Model file for the job. Use its own axes, mm. A direction names the side the tool comes from. Give positions to 0.01 mm unless a question says otherwise; leave off trailing zeros. Loops run counter-clockwise (first coordinate to the right, second up) from the corner with the lowest first, then second, coordinate; pieces in that order, holes last. Notation, with made-up numbers: (-3, 70.5) - (54, 70.5) arc R19 cw to (54, 82.5) - close; hole circle Ø8 at (-25.5, 33). An arc over 180 degrees is marked (long way). Answer as CSV lines item,"result". Start each with the question number.
Item 1: Pull direction Y, two halves, no side cores. Call faces 1 (the flat face through (-20.3, 0, 7)), 2 (the flat face through (0, 15.4, 26)), 3 (the flat face through (0.148, -6.034, 30.325)): pulls with the +Y half, pulls with the -Y half, needs draft (parallel to the pull), parting line crosses it, or undercut.
Item 2: Saw through at A-A on z = 36. Give the cut face in (x, y).
Item 3: Drill centre lines: L1, parallel to X at y = -4, z = 8; L2, parallel to Y at x = 0.5, z = 28.5; L3, parallel to Z at x = 3, y = -5. Where is each one in solid material? Low to high. Write a range as from..to.
Item 4: Saw through at D-D on x = 7.5. Give the cut face in (y, z).
Item 5: Pin check, flat tips, straight feed: pin 1 (1.7 mm diameter, centred on x = -18, z = 15.5, fed in from +Y); pin 2 (1.5 mm diameter, centred on y = 5.5, z = 34.5, fed in from -X); pin 3 (10 mm diameter, centred on x = 12.5, z = 30.5, fed in from +Y); pin 4 (2 mm diameter, centred on y = -9, z = 23, fed in from +X). Stop position of each tip, or through.
Item 6: Tool access for faces 4 (the flat face through (18, -9.4, 8)), 5 (the flat face through (-18, 0, 0)), 6 (the flat face through (-10.6, 0, 30)): list every direction of +Z, -Z, +X, -X, +Y, -Y with a clear straight run to the whole face (end or side of a thin tool).
Item 7: Saw through at B-B on z = 7.5. Give the cut face in (x, y), plus the area to 3 significant figures.
Autodesk Inventor part; units mm, degrees
ref_plane "YZ Plane" through (0, 0, 0) normal (1, 0, 0) x (0, 1, 0)
ref_plane "XZ Plane" through (0, 0, 0) normal (0, 1, 0) x (-1, 0, 0)
ref_plane "XY Plane" through (0, 0, 0) normal (0, 0, 1) x (1, 0, 0)
sketch "Sketch1" plane through (0, 0, 0) normal (0, 0, 1) x (1, 0, 0)
  line L0 (-20.3, 9.4) -> (20.3, 9.4)
  line L1 (20.3, 9.4) -> (20.3, -9.4)
  line L2 (20.3, -9.4) -> (-20.3, -9.4)
  line L3 (-20.3, -9.4) -> (-20.3, 9.4)
  line L4 (-14.7, 9.4) -> (14.7, 9.4)
  line L5 (14.7, 9.4) -> (14.7, -9.4)
  line L6 (14.7, -9.4) -> (-14.7, -9.4)
  line L7 (-14.7, -9.4) -> (-14.7, 9.4)
  point P0 (0, 0)
  point P1 (14.7, 9.4)
  dimension "d0" = 29.4
  dimension "d1" = 18.8
  dimension "d2" = 9.4
  dimension "d3" = 14.7
  dimension "d4" = 5.6
  dimension "d5" = 5.6
extrude "Extrusion1" add sketch "Sketch1" along normal blind 18
extrude "Extrusion2" cut sketch "Sketch1" along normal blind 10 contours L0 L5 L2 L7
sketch "Sketch2" plane through (0, 0, 18) normal (0, 0, 1) x (1, 0, 0)
  line L0 (10.6, 0) -> (-10.6, 12.2398)
  line L1 (-10.6, 12.2398) -> (-10.6, -12.2398)
  line L2 (14.7, 9.4) -> (-14.7, 9.4)
  line L3 (-10.6, -12.2398) -> (10.6, 0)
  line L4 (-20.3, 9.4) -> (-20.3, -9.4)
  line L5 (14.7, -9.4) -> (14.7, 9.4)
  line L6 (-14.7, 9.4) -> (-14.7, -9.4)
  line L7 (14.7, -9.4) -> (-14.7, -9.4)
  line L8 (-14.7, -9.4) -> (-14.7, -15.4)
  line L9 (-14.7, -15.4) -> (14.7, -15.4)
  line L10 (14.7, -15.4) -> (14.7, -9.4)
  line L11 (14.7, 9.4) -> (-14.7, 9.4)
  line L12 (-14.7, 9.4) -> (-14.7, 15.4)
  line L13 (-14.7, 15.4) -> (14.7, 15.4)
  line L14 (14.7, 15.4) -> (14.7, 9.4)
  point P0 (0, 0)
  point P1 (-10.6, 0)
  point P2 (0, -6.1199)
  point P3 (0, 6.1199)
  point P4 (-14.7, 9.4)
  point P5 (-14.7, -9.4)
  point P6 (-5.6813, -9.4)
  point P7 (-10.6, -9.4)
  point P8 (-10.6, 9.4)
  point P9 (-5.6813, 9.4)
  dimension "d17" = 21.2
  dimension "d18" = 0
  dimension "d19" = 21.2
  dimension "d20" = 21.2
  dimension "d21" = 10.6
  dimension "d25" = 6
  dimension "d26" = 6
  dimension "d27" = 0
  dimension "d28" = 0
extrude "Extrusion3" add sketch "Sketch2" along normal blind 10 and the other way blind 8 contours L0 L2 L5 L7 L3 | L0 L1 L2 L12 L13 L14 | L7 L10 L9 L8 L1 L3 | L1 L7 L6 L2
extrude "Extrusion4" add sketch "Sketch2" against normal blind 8 contours L2 L1 L0 | L3 L1 L7
chamfer "Chamfer1" distance 6 angle 45 4 edges at (-14.7, 15.4, 19) (-14.7, -15.4, 19) (14.7, -15.4, 19) (14.7, 15.4, 19)
fillet "Fillet1" radius 3 4 edges at (14.7, 0, 18) (-14.7, 0, 18) (-20.3, 0, 18) (20.3, 0, 18)
sketch "Sketch4" plane through (0, 0, 28) normal (0, 0, 1) x (1, 0, 0)
  line L0 (8.7, 15.4) -> (14.7, 9.4)
  line L1 (8.7, 15.4) -> (-8.7, 15.4)
  line L2 (-14.7, 9.4) -> (-8.7, 15.4)
  line L3 (-14.7, 9.4) -> (-14.7, -9.4)
  line L4 (-8.7, -15.4) -> (-14.7, -9.4)
  line L5 (-8.7, -15.4) -> (8.7, -15.4)
  line L6 (14.7, -9.4) -> (8.7, -15.4)
  line L7 (14.7, -9.4) -> (14.7, 9.4)
  line L8 (-10.6, 12.2398) -> (10.6, 0)
  line L9 (10.6, 0) -> (-10.6, -12.2398)
  line L10 (-10.6, -12.2398) -> (-10.6, 12.2398)
  point P0 (0, 0)
extrude "Extrusion5" add sketch "Sketch4" along normal blind 15
equation "\"d5\" = d4"
properties part number "CameraSupportTemp"
Responses:
1,face 1,"needs draft"
1,face 2,"pulls with the +Y half"
1,face 3,"undercut"
2,outline,"(-14.7, -9.4) - (-8.7, -15.4) - (8.7, -15.4) - (14.7, -9.4) - (14.7, 9.4) - (8.7, 15.4) - (-8.7, 15.4) - (-14.7, 9.4) - close; hole (-10.6, -12.24) - (10.6, 0) - (-10.6, 12.24) - close"
3,L1,"-20.3..-14.7, 14.7..20.3"
3,L2,"-15.4..-5.83, 5.83..15.4"
3,L3,"10..43"
4,outline,"(-15.4, 10) - (15.4, 10) - (15.4, 43) - (1.79, 43) - (1.79, 18) - (-1.79, 18) - (-1.79, 43) - (-15.4, 43) - close"
5,pin 1,"y = 9.4"
5,pin 2,"x = -14.7"
5,pin 3,"y = 15.4"
5,pin 4,"x = 14.7"
6,face 4,"+Z, -Z, +X, -Y"
6,face 5,"-Z, +X, -X, +Y, -Y"
6,face 6,"+Z"
7,outline,"(-20.3, -9.4) - (-14.7, -9.4) - (-14.7, 9.4) - (-20.3, 9.4) - close; (14.7, -9.4) - (20.3, -9.4) - (20.3, 9.4) - (14.7, 9.4) - close"
7,area,"211 mm2"
